```python
from build123d import *

# Parameters (mm, degrees)
F0_W      = 101.6
F0_H      = 19.05
F1_DEPTH  = 254
F2_W      = 6.35
F2_H      = 254
F3_DEPTH  = 2.54
F4_W      = 101.6
F4_H      = 6.35
F5_DEPTH  = 2.54
F6_W      = 101.6
F6_H      = 6.35
F7_DEPTH  = 2.54
F8_W      = 101.6
F8_H      = 6.35
F9_DEPTH  = 2.54
F10_R     = 6.35
F11_DEPTH = 0.254
F12_W     = 19.05
F12_H     = 254
F13_DEPTH = 20.32
F15_DEPTH = 2.54


with BuildPart() as f1:
    # F0 (on Top) → F1 (new body)
    with BuildSketch(Plane.XY):
        Rectangle(F0_W, F0_H)
    extrude(amount=F1_DEPTH)

    # F2 (on face) → F3 (join)
    with BuildSketch(Plane.XZ.offset(9.525)):
        with Locations((0, 127)):
            Rectangle(F2_W, F2_H)
    extrude(amount=F3_DEPTH)

    # F4 (on face) → F5 (join)
    with BuildSketch(Plane.XZ.offset(9.525)):
        with Locations((0, 127)):
            Rectangle(F4_W, F4_H)
    extrude(amount=F5_DEPTH)

    # F6 (on face) → F7 (join)
    with BuildSketch(Plane.XZ.offset(9.525)):
        with Locations((0, 192.0875)):
            Rectangle(F6_W, F6_H)
    extrude(amount=F7_DEPTH)

    # F8 (on face) → F9 (join)
    with BuildSketch(Plane.XZ.offset(9.525)):
        with Locations((0, 61.9125)):
            Rectangle(F8_W, F8_H)
    extrude(amount=F9_DEPTH)

    # F10 (on face) → F11 (join)
    with BuildSketch(Plane.XZ.offset(9.525)):
        with Locations((26.9875, 159.54375)):
            Circle(F10_R)
    extrude(amount=F11_DEPTH)

    # F12 (on face) → F13 (join)
    with BuildSketch(Plane(origin=(-50.8, 0, 0), x_dir=(0, -1, 0), z_dir=(-1, 0, 0))):
        with Locations((0, 127)):
            Rectangle(F12_W, F12_H)
    extrude(amount=F13_DEPTH)

    # F14 (on face) → F15 (join)
    with BuildSketch(Plane.XZ.offset(9.525)):
        Polygon((-50.8, 123.825), (-50.8, 127), (-50.8, 128.689587), (-50.8, 254), (-57.15, 254), (-57.15, 0), (-50.8, 0), align=None)
    extrude(amount=F15_DEPTH)


solid = f1.part
```
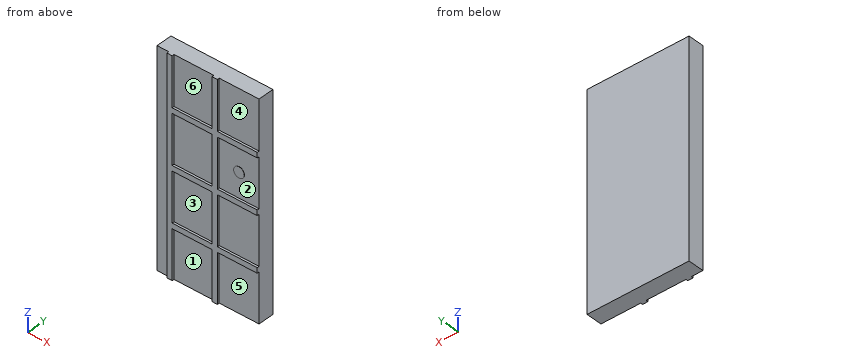
Input: part model. Units: mm. Frame: model coordinates. Face numbers are marked on the shaded views. A direction names the side the tool comes from. Coordinates: 2 decimals unless noted, no trailing zeros. Loops run counter-clockwise (first coordinate to the right, second up) from the corner with the lowest first, then second, coordinate; pieces in that order, holes last.
Q1. Line query: line 1 along Y through (x, z) = (-26, 173.5) (3 decimals). Output: solid intervals per line, ascending.
Results are:
line 1: y = -9.525 to 9.525
Q2. Section B-B, the plane x = 13. Return the cut outline in (y, z) (1 decimal), and give its area (3 significant figures).
Results are:
outline: (-12.1, 58.7) - (-9.5, 58.7) - (-9.5, 0) - (9.5, 0) - (9.5, 254) - (-9.5, 254) - (-9.5, 195.3) - (-12.1, 195.3) - (-12.1, 188.9) - (-9.5, 188.9) - (-9.5, 130.2) - (-12.1, 130.2) - (-12.1, 123.8) - (-9.5, 123.8) - (-9.5, 65.1) - (-12.1, 65.1) - close
area: 4,890 mm2
Q3. Mould query, pull axis Z, two halves, no side actions, for the marked faces 1 and 2. Classes: +Z half, -Z half, draft (parallel to the pull), parting line (faces both ways), or undercut.
Results are:
face 1: draft
face 2: undercut
Q4. Contact query for flat-ended pins moving along their axis: pin 1 (1 mm diameter, centred on x = 38, z = 82, fed in from -Y) (3 decimals); pin 2 (1.3 mm diameter, centred on x = -37, y = -11, fed in from -Z); pin 3 (0.8 mm diameter, centred on y = -11, z = 235, fed in from -X). Output: stop coordinate, or through.
Results are:
pin 1: stops at y = -9.525
pin 2: stops at z = 58.74
pin 3: stops at x = -57.15
Q5. Section A-A, the plane z = 25.5. Return the cut outline in (x, y) (3 decimals).
Results are:
outline: (-71.12, -9.525) - (-57.15, -9.525) - (-57.15, -12.065) - (-50.8, -12.065) - (-50.8, -9.525) - (-3.175, -9.525) - (-3.175, -12.065) - (3.175, -12.065) - (3.175, -9.525) - (50.8, -9.525) - (50.8, 9.525) - (-71.12, 9.525) - close
Q6. Set-up query: the marked faces 3, 4, 5 and 6. Return all of +Z, -Z, +X, -X, +Y, -Y with unobstructed straight access to the full face (end or side cutting, diameter ignored); none if empty.
Results are:
face 3: -Y
face 4: +Z, +X, -Y
face 5: -Z, +X, -Y
face 6: +Z, -Y
